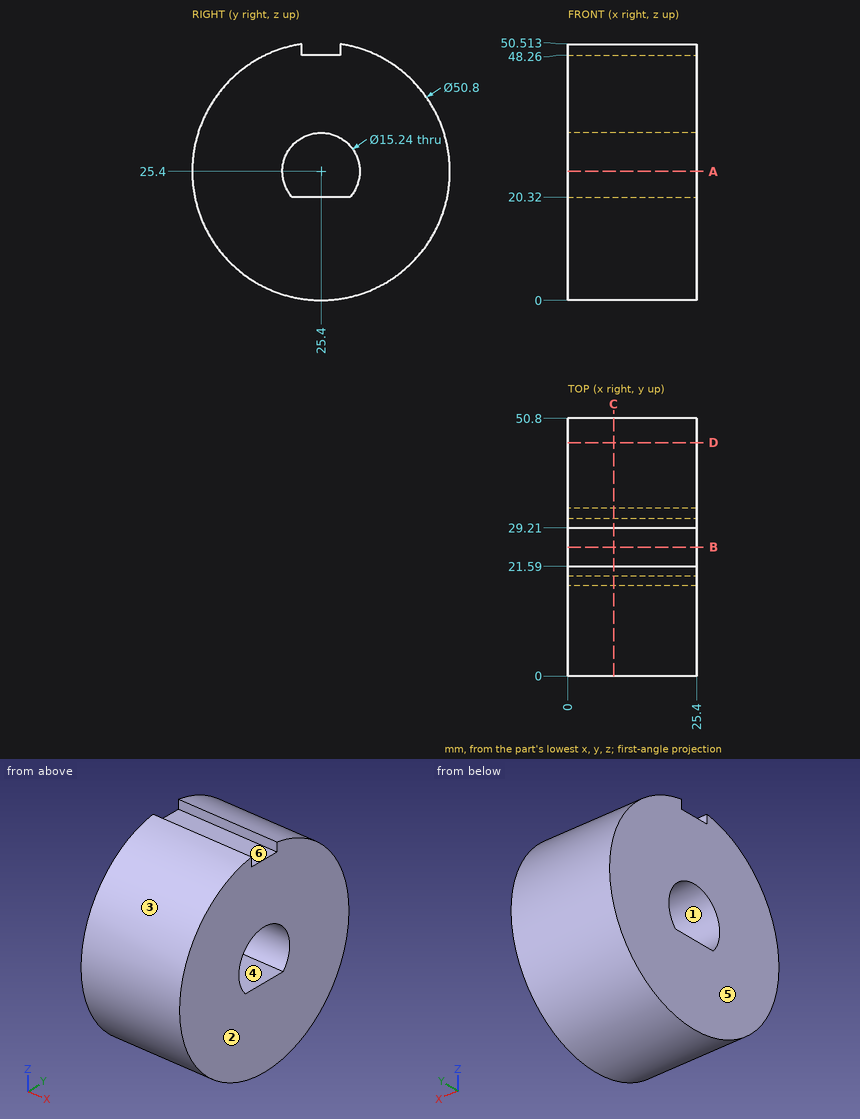
Geometry check sheet. Reference: drawing and pictorial views, mm from the part's lowest x, y, z. A direction names the side the tool comes from. Round coordinates to 2 decimals unless told otherwise and drop trailing zeros. Loops run counter-clockwise (first coordinate to the right, second up) from the corner with the lowest first, then second, coordinate; pieces in that order, holes last. Notation, with made-up numbers: (69, -30) -> (87, -30) arc R24 cw to (87, -20) -> close; hole circle Ø7 at (47.25, -18.5). An arc over 180 degrees is marked (long way). Answer as a JSON object with one key per item and string values.
Q1. Access from +Z, -Z, +X, -X, +Y, -Y to the whole of each face (thin tool, end or side, straight path). Record for the marked faces 4, 5 and 6.
Data:
{"face 4": "+X, -X", "face 5": "+Z, -Z, -X, +Y, -Y", "face 6": "+Z, +X, -X"}
Q2. Section check D-D (y = 46). Record the boundary of the cut face in (x, z).
Data:
{"outline": "(0, 10.54) -> (25.4, 10.54) -> (25.4, 40.26) -> (0, 40.26) -> close"}
Q3. Section check C-C (x = 9). Record the boundary of the cut face in (y, z).
Data:
{"outline": "(21.59, 48.26) -> (21.59, 50.51) arc R25.4 ccw (long way) to (29.21, 50.51) -> (29.21, 48.26) -> close; hole (19.72, 20.32) -> (31.08, 20.32) arc R7.62 ccw (long way) to start"}
Q4. Scan lines: line 1 (Y direction, x = 18.5, z = 25); line 2 (Z direction, x = 9.5, y = 25.4); line 3 (Y direction, x = 21.5, z = 22). Record each from-to range of solid material in increasing order. Write a range as from..to.
Data:
{"line 1": "y = 0..17.79, 33.01..50.8", "line 2": "z = 0..20.32, 33.02..48.26", "line 3": "y = 0.23..18.58, 32.22..50.57"}
Q5. Draft check along Y on the marked faces 1, 2 and 3. Enter one of: pulls with the +Y half, pulls with the -Y half, needs draft (parallel to the pull), parting line crosses it, or undercut.
Data:
{"face 1": "undercut", "face 2": "needs draft", "face 3": "parting line crosses it"}
Q6. Go/stop test with flat-tipped pins: P1, Ø4, axis at x = 21.5, y = 35.5, coming from the +Z side; P2, Ø1.1, axis at x = 7.5, z = 49.5, coming from the +Y side (1 decimal); P3, Ø1.5, axis at x = 19, y = 13, coming from the -Z side. Record where each tip stops, or that it passes through.
Data:
{"P1": "stops at z = 49.47", "P2": "stops at y = 34.9", "P3": "stops at z = 2.83"}
Q7. Section check B-B (y = 25.4). Record the boundary of the cut face in (x, z), then the cut area to 3 significant figures.
Data:
{"outline": "(0, 0) -> (25.4, 0) -> (25.4, 20.32) -> (0, 20.32) -> close; (0, 33.02) -> (25.4, 33.02) -> (25.4, 48.26) -> (0, 48.26) -> close", "area": "903 mm2"}
Q8. Section check A-A (z = 25.4). Record the boundary of the cut face in (x, y), then the cut area to 3 significant figures.
Data:
{"outline": "(0, 0) -> (25.4, 0) -> (25.4, 17.78) -> (0, 17.78) -> close; (0, 33.02) -> (25.4, 33.02) -> (25.4, 50.8) -> (0, 50.8) -> close", "area": "903 mm2"}
